Geometry: final body of the model. Coordinates: model frame, mm. Face numbers are marked on the shaded views. A direction names the side the tool comes from. Coordinates: 2 decimals unless noted, no trailing zeros. Write each loop counter-clockwise with the first axis right and the second up, starting at its lowest first coordinate (ties: lowest second). Pieces come first, ordered by that corner, then holes. Notation, with made-up numbers: (82.25, 11) -> (138.25, 11) arc R6 ccw to (138.25, 18) -> close; hole circle Ø5 at (-22, 46.25). An arc over 180 degrees is marked (long way). Answer as a JSON object with one key per item and string values. Group by question number.
```python
from build123d import *

# Parameters (mm, degrees)
EXTRUDE_1_DEPTH     = 60
CUT_EXTRUDE_1_DEPTH = 10
CUT_EXTRUDE_2_DEPTH = 10
SKETCH_4_R          = 40
CUT_EXTRUDE_3_DEPTH = 20
SKETCH_5_R          = 4
CUT_EXTRUDE_4_DEPTH = 5


with BuildPart() as part:
    # 草图1 → 凸台-拉伸1 (new body)
    with BuildSketch(Plane.XY):
        with BuildLine():
            Line((56.568542495, -20), (76.568542495, -20))
            Line((76.568542495, -20), (76.568542495, 20))
            Line((76.568542495, 20), (56.568542495, 20))
            ThreePointArc((56.568542495, 20), (-60, 0), (56.568542495, -20))
        make_face()
    extrude(amount=EXTRUDE_1_DEPTH)

    # 草图2 → 切除-拉伸1 (cut)
    with BuildSketch(Plane(origin=(0, 0, 0), x_dir=(-1, 0, 0), z_dir=(0, 0, -1))):
        with BuildLine():
            Line((-76.568542495, 20), (-76.568542495, -20))
            Line((-76.568542495, -20), (-56.568542495, -20))
            ThreePointArc((-56.568542495, -20), (-60, 0), (-56.568542495, 20))
            Line((-56.568542495, 20), (-76.568542495, 20))
        make_face()
    extrude(amount=-CUT_EXTRUDE_1_DEPTH, mode=Mode.SUBTRACT)

    # 草图3 → 切除-拉伸2 (cut)
    with BuildSketch(Plane.XY.offset(60)):
        with BuildLine():
            Line((76.568542495, 20), (76.568542495, -20))
            Line((76.568542495, -20), (56.568542495, -20))
            ThreePointArc((56.568542495, -20), (60, 0), (56.568542495, 20))
            Line((56.568542495, 20), (76.568542495, 20))
        make_face()
    extrude(amount=-CUT_EXTRUDE_2_DEPTH, mode=Mode.SUBTRACT)

    # 草图4 → 切除-拉伸3 (cut)
    with BuildSketch(Plane(origin=(0, 0, 0), x_dir=(-1, 0, 0), z_dir=(0, 0, -1))):
        Circle(SKETCH_4_R)
    extrude(amount=-CUT_EXTRUDE_3_DEPTH, mode=Mode.SUBTRACT)

    # 草图5 → 切除-拉伸4 (cut)
    with BuildSketch(Plane(origin=(76.568542495, 0, 0), x_dir=(0, 0, -1), z_dir=(1, 0, 0))):
        with Locations((-17.5, 12.5)):
            Circle(SKETCH_5_R)
        with Locations((-17.5, -12.5)):
            Circle(SKETCH_5_R)
        with Locations((-42.5, -12.5)):
            Circle(SKETCH_5_R)
        with Locations((-42.5, 12.5)):
            Circle(SKETCH_5_R)
    extrude(amount=-CUT_EXTRUDE_4_DEPTH, mode=Mode.SUBTRACT)


solid = part.part
```
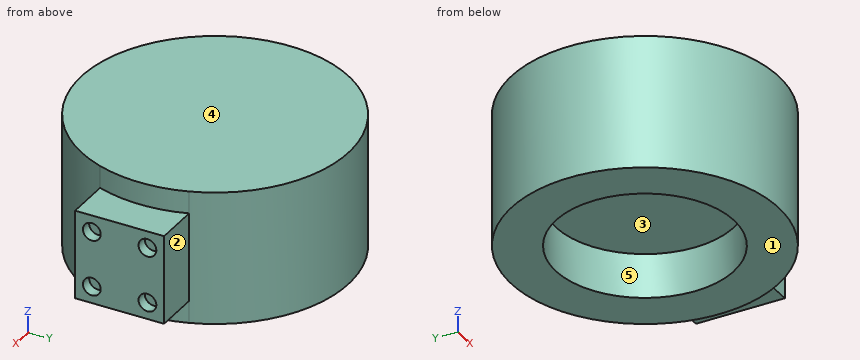
Item 1: Ray query, L1, parallel to Y at x = 75, z = 42.5; L2, parallel to Z at x = 75, y = -12; L3, parallel to Z at x = 1.5, y = 34. Return the intervals inside material, ascending. Write a range as [from, to].
Item 2: Section C-C on y = 0. Output: boundary loops of the cut face in (x, z), then the cut area to 3 significant figures.
Item 3: Set-up query: the marked faces 4 and 5. Return all of +Z, -Z, +X, -X, +Y, -Y with unobstructed straight access to the full face (end or side cutting, diameter ignored); none if empty.
Item 4: Section B-B on x = 0. Output: boundary loops of the cut face in (y, z).
Item 5: Section A-A on z = 17.5. Output: boundary loops of the cut face in (x, y).
Item 6: Contact query for flat-ended pins moving along their axis: pin 1 (5 mm diameter, centred on y = 12.5, z = 17.5, fed in from +X); pin 2 (16 mm diameter, centred on x = 69, y = -9.5, fed in from +Z); pin 3 (3 mm diameter, centred on x = 53, z = 10, fed in from +Y). Output: stop coordinate, or through.
Item 7: Section D-D on z = 42. Output: boundary loops of the cut face in (x, y).
Item 8: Mould query, pull axis Y, two halves, no side actions, for the marked faces 1, 2 and 3. Classes: +Y half, -Y half, draft (parallel to the pull), parting line (faces both ways), or undercut.
Answer sheet:
{
 "1": {"L1": "y = [-20, -16.5], [-8.5, 8.5], [16.5, 20]", "L2": "z = [10, 13.53], [21.47, 38.53], [46.47, 50]", "L3": "z = [20, 60]"},
 "2": {"outline": "(-60, 0) -> (-40, 0) -> (-40, 20) -> (40, 20) -> (40, 0) -> (60, 0) -> (60, 10) -> (76.57, 10) -> (76.57, 50) -> (60, 50) -> (60, 60) -> (-60, 60) -> close", "area": "6,260 mm^2"},
 "3": {"face 4": "+Z, +X, -X, +Y, -Y", "face 5": "-Z"},
 "4": {"outline": "(-60, 0) -> (-40, 0) -> (-40, 20) -> (40, 20) -> (40, 0) -> (60, 0) -> (60, 60) -> (-60, 60) -> close"},
 "5": {"outline": "(56.57, -20) -> (76.57, -20) -> (76.57, -16.5) -> (71.57, -16.5) -> (71.57, -8.5) -> (76.57, -8.5) -> (76.57, 8.5) -> (71.57, 8.5) -> (71.57, 16.5) -> (76.57, 16.5) -> (76.57, 20) -> (56.57, 20) arc R60 ccw (long way) to start; hole circle Ø80 at (0, 0)"},
 "6": {"pin 1": "stops at x = 71.57", "pin 2": "stops at z = 50", "pin 3": "stops at y = 30.79"},
 "7": {"outline": "(56.57, -20) -> (76.57, -20) -> (76.57, -16.47) -> (71.57, -16.47) -> (71.57, -8.53) -> (76.57, -8.53) -> (76.57, 8.53) -> (71.57, 8.53) -> (71.57, 16.47) -> (76.57, 16.47) -> (76.57, 20) -> (56.57, 20) arc R60 ccw (long way) to start"},
 "8": {"face 1": "draft", "face 2": "+Y half", "face 3": "undercut"}
}
